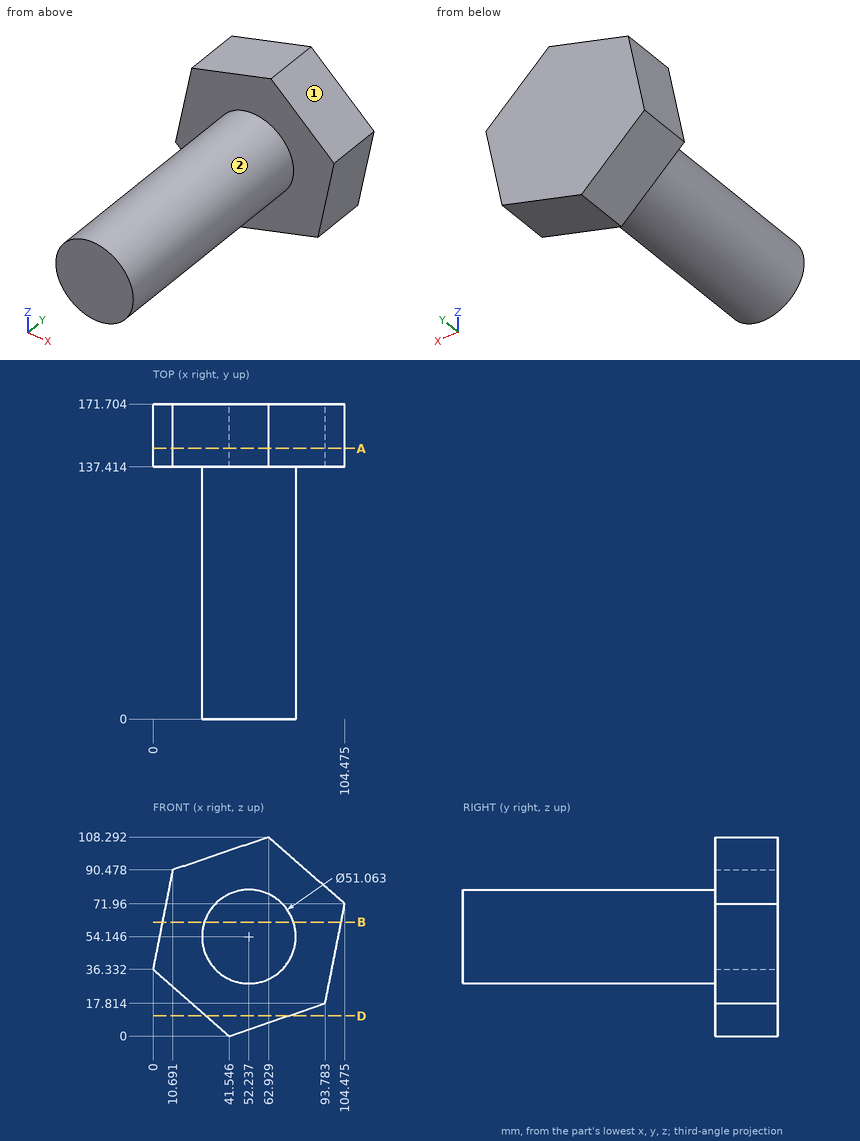
Could you check a few things on this drawing? It's one solid part, dimensions in mm from its lowest x, y, z. A direction names the side the tool comes from. Give positions to 0.01 mm unless a question says otherwise; leave off trailing zeros. Order: outer loops, then holes, each group sorted by start corner. A loop starts at its lowest first (then second) coordinate and runs counter-clockwise, first axis right, second up. Notation, with made-up numbers: (80, 50) - (137, 50) arc R22 cw to (137, 74) - close; hole circle Ø2 at (-26.5, 37.5). An arc over 180 degrees is marked (long way). One line per item, written item: value. Start each with the question number.
1. Imagine slicing it at B-B on z = 62. List the corners of the cut face in (x, y) for me (1 decimal).
2. For the marked faces 1 and 2, which set-ups out of +Z, -Z, +X, -X, +Y, -Y let a thin tool reach every point of the face, with its end or its side?
3. If I drill on probe 1 along Y at (x, z) = (27, 88); probe 2 along Z at (x, y) = (67, 160); probe 3 along Z at (x, y) = (14, 163) (1 decimal), over which ranges is the centre line in solid material (lowest first)?
4. For P1, Ø2, axis at x = 30.5, y = 44.5, coming from the -Z side; P2, Ø12, axis at y = 127, z = 35.5, coming from the +X side; P3, Ø2, axis at y = 117, z = 54.5, coming from the -X side, each with a flat end and sliding along its axis, tell me the tip position at first contact or that it passes through.
5. Imagine slicing it at A-A on y = 147.5. List the corners of the cut face in (x, z) for me (1 decimal), plus the area to 3 significant figures.
6. Imagine slicing it at D-D on z = 11. List the corners of the cut face in (x, y) for me, plus the area to 3 significant figures.
Values:
1. outline: (5.1, 137.4) - (27.9, 137.4) - (27.9, 0) - (76.5, 0) - (76.5, 137.4) - (102.5, 137.4) - (102.5, 171.7) - (5.1, 171.7) - close
2. face 1: +Z, +X, +Y, -Y
2. face 2: -Y
3. probe 1: 137.41 to 171.7
3. probe 2: 8.68 to 104.73
3. probe 3: 24.1 to 91.6
4. P1: z = 39.25
4. P2: x = 74.42
4. P3: x = 26.71
5. outline: (0, 36.3) - (41.5, 0) - (93.8, 17.8) - (104.5, 72) - (62.9, 108.3) - (10.7, 90.5) - close
5. area: 7,910 mm²
6. outline: (28.97, 137.41) - (73.8, 137.41) - (73.8, 171.7) - (28.97, 171.7) - close
6. area: 1,540 mm²
